Build history of the part. All positions in model axes, mm. Face numbers are marked on the shaded views. Give positions to 0.01 mm unless a question says otherwise; leave off trailing zeros. Order: outer loops, then holes, each group sorted by start corner. A loop starts at its lowest first (then second) coordinate and runs counter-clockwise, first axis right, second up. Notation, with made-up numbers: (74, 16.25) -> (120, 16.25) arc R35 ccw to (120, 49.25) -> close; hole circle Ø8 at (71, -13.5). An arc over 180 degrees is marked (long way). One line per item, written item: value. Start each with the question number.
(1) Probe line 1 (Y direction, x = 4, z = 8); line 2 (X direction, y = 4.55, z = 0); line 3 (X direction, y = -12.6, z = 0). List the from-to ranges inside material, lowest first.
(2) Saw through at C-C on z = 0. Count the separate pieces of the cut face and the enclosed holes in it, plus the area to 3 significant figures.
(3) Pin check, flat tips, straight feed: pin 1 (14.5 mm diameter, centred on x = 0, z = 0, fed in from +Y); pin 2 (14.5 mm diameter, centred on x = -2.5, z = 2, fed in from +Y); pin 3 (1.5 mm diameter, centred on y = -11.5, z = 11, fed in from -X); pin 4 (2 mm diameter, centred on x = -11, y = -11, fed in from +Z). Stop position of each tip, or through.
(4) Two-plate mould, pull along X, no slides. Class the marked faces 1, 2 and 3: +X half, -X half, draft (parallel to the pull), parting line (faces both ways), or undercut.
(5) Saw through at B-B on y = 9.5. Give the cut face in (x, z), plus the area to 3 significant figures.
(6) Saw through at A-A on y = -7.25. Give the cut face in (x, z).
```python
from build123d import *

# Parameters (mm, degrees)
ESBO_O4_W                        = 2.25
ESBO_O4_H                        = 16
F_4_5_4_5_DIAMETER_HOLE2_D       = 4.5
F_4_5_4_5_DIAMETER_HOLE2_DEPTH   = 18
F_4_5_4_5_DIAMETER_HOLE2_TIP     = 1.351936393
ESBO_O12_R                       = 16
ESBO_O12_R_2                     = 9
RESSALTO_EXTRUS_O1_DEPTH         = 1
CHANFRO1_SIZE                    = 0.5
CHANFRO2_SIZE                    = 0.25
FURO_DE_DI_METRO_4_5_4_5_2_D     = 4.5
FURO_DE_DI_METRO_4_5_4_5_2_DEPTH = 8
FURO_DE_DI_METRO_4_5_4_5_2_TIP   = 1.351936393


# Read off the part's stored shape, not the designer's step: PadrãoCircular5
with BuildPart() as part:
    # Esboço1 → Revolução1 (revolve)
    with BuildSketch(Plane.XY, mode=Mode.PRIVATE) as revolu_o1_sk:
        Polygon((3, -14), (16, -14), (16, 10), (8, 10), (8, 8.5), (9, 8.5), (9, 6.5), (8, 6.5), (8, 5), (9.5, 5), (9.5, 3), (9, 3), (9, -3), (9.5, -3), (9.5, -5), (8, -5), (8, -6.5), (9, -6.5), (9, -8.5), (8, -8.5), (8, -10), (3, -10), align=None)
    revolve(revolu_o1_sk.sketch.rotate(Axis((0, -14, 0), (0, 1, 0)), 90), axis=Axis((0, -14, 0), (0, 1, 0)))

    # Esboço4 → Furo de diâmetro Ø4.5 (4.5)1 (revolve, cut)
    with BuildSketch(Plane(origin=(16, 0, 0), x_dir=(0, 0, -1), z_dir=(0, 1, 0))):
        with Locations((1.125, 8)):
            Rectangle(ESBO_O4_W, ESBO_O4_H)
    revolve(axis=Axis((22.35, 0, 0), (-1, 0, 0)), mode=Mode.SUBTRACT)

    # Ø4.5 (4.5) Diameter Hole2
    with Locations(Plane(origin=(-13.856406461, 0, -8), x_dir=(0, -1, 0), z_dir=(-0.8660254037844364, 0, -0.5000000000000041))):
        with Locations((0, 0)):
            Hole(F_4_5_4_5_DIAMETER_HOLE2_D / 2, depth=F_4_5_4_5_DIAMETER_HOLE2_DEPTH)
            with Locations((0, 0, -(F_4_5_4_5_DIAMETER_HOLE2_DEPTH + F_4_5_4_5_DIAMETER_HOLE2_TIP / 2))):  # 118° drill point
                Cone(0, F_4_5_4_5_DIAMETER_HOLE2_D / 2, F_4_5_4_5_DIAMETER_HOLE2_TIP, mode=Mode.SUBTRACT)

    # Esboço12 → Ressalto-extrusão1 (add)
    with BuildSketch(Plane(origin=(0, 10, 0), x_dir=(1, 0, 0), z_dir=(0, 1, 0))):
        with Locations(Location((0, 0, 0), (0, 0, 90))):
            Circle(ESBO_O12_R)
        with Locations(Location((0, 0, 0), (0, 0, 90))):
            Circle(ESBO_O12_R_2, mode=Mode.SUBTRACT)
    extrude(amount=RESSALTO_EXTRUS_O1_DEPTH)

    # Esboço13 → Furo roscado de M3x0.51 (revolve, cut)
    with BuildSketch(Plane(origin=(11.328847338, 11, -5.282728272), x_dir=(0, 0, 1), z_dir=(1, 0, 0))):
        Polygon((0, 0), (0, 10.751075774), (1.25, 10), (1.25, 0), align=None)
    revolve(axis=Axis((11.328847338, 17.35, -5.282728272), (0, -1, 0)), mode=Mode.SUBTRACT)

    # PadrãoCircular5 outline → PadrãoCircular5 (revolve, cut)
    with BuildSketch(Plane(origin=(5.282728272, 0, 11.328847338), x_dir=(1, 0, 0), z_dir=(0, 0, 1))):
        Polygon((0, 11), (0, 0.248924226), (1.25, 1), (1.25, 11), align=None)
    revolve(axis=Axis((5.282728272, 0, 11.328847338), (0, 1, 0)), mode=Mode.SUBTRACT)

    # Padr_oCircular5 2 outline → Padr_oCircular5 2 (revolve, cut)
    with BuildSketch(Plane(origin=(-11.328847338, 0, 5.282728272), x_dir=(1, 0, 0), z_dir=(0, 0, 1))):
        Polygon((0, 11), (0, 0.248924226), (1.25, 1), (1.25, 11), align=None)
    revolve(axis=Axis((-11.328847338, 0, 5.282728272), (0, 1, 0)), mode=Mode.SUBTRACT)

    # Padr_oCircular5 3 outline → Padr_oCircular5 3 (revolve, cut)
    with BuildSketch(Plane(origin=(-5.282728272, 0, -11.328847338), x_dir=(1, 0, 0), z_dir=(0, 0, 1))):
        Polygon((0, 11), (0, 0.248924226), (1.25, 1), (1.25, 11), align=None)
    revolve(axis=Axis((-5.282728272, 0, -11.328847338), (0, 1, 0)), mode=Mode.SUBTRACT)

    # Chanfro1
    chanfro1_edges = [part.edges().sort_by_distance(p)[0] for p in [
        (0, -10, 3),
    ]]
    chamfer(chanfro1_edges, length=CHANFRO1_SIZE)

    # Chanfro2
    chanfro2_edges = [part.edges().sort_by_distance(p)[0] for p in [
        (0, 11, 9),
    ]]
    chamfer(chanfro2_edges, length=CHANFRO2_SIZE)

    # Furo de diâmetro Ø4.5 (4.5)2
    with Locations(Plane(origin=(-16, 0, 0), x_dir=(0, 0, -1), z_dir=(-1, 0, 0))):
        with Locations((0, 0)):
            Hole(FURO_DE_DI_METRO_4_5_4_5_2_D / 2, depth=FURO_DE_DI_METRO_4_5_4_5_2_DEPTH)
            with Locations((0, 0, -(FURO_DE_DI_METRO_4_5_4_5_2_DEPTH + FURO_DE_DI_METRO_4_5_4_5_2_TIP / 2))):  # 118° drill point
                Cone(0, FURO_DE_DI_METRO_4_5_4_5_2_D / 2, FURO_DE_DI_METRO_4_5_4_5_2_TIP, mode=Mode.SUBTRACT)


solid = part.part
```
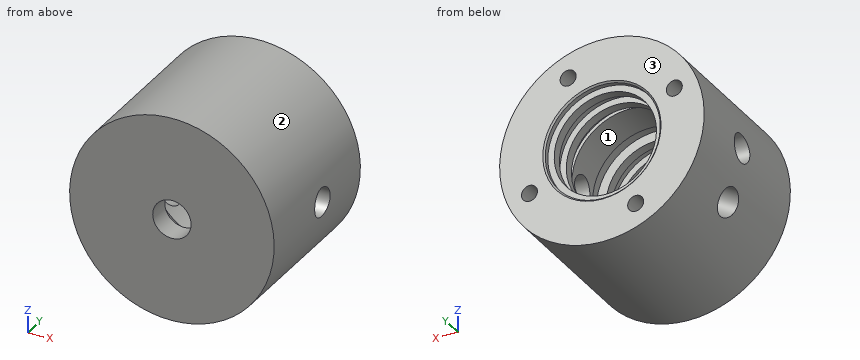
Results below:
1. line 1: y = -14 to -8.5, -6.5 to -5, 5 to 6.5, 8.5 to 10
1. line 2: x = -16 to -9.5, 9.5 to 16
1. line 3: x = -16 to -3, 3 to 16
2. separate pieces: 4
2. enclosed holes: 0
2. area: 343 mm²
3. pin 1: stops at y = -10
3. pin 2: stops at y = 11
3. pin 3: stops at x = -12.29
3. pin 4: stops at z = 12.49
4. face 1: undercut
4. face 2: parting line
4. face 3: draft
5. outline: circle Ø32 at (0, 0); hole circle Ø2.5 at (-11.33, 5.28); hole circle Ø16 at (0, 0); hole circle Ø2.5 at (-5.28, -11.33); hole circle Ø2.5 at (5.28, 11.33); hole circle Ø2.5 at (11.33, -5.28)
5. area: 584 mm²
6. outline: circle Ø32 at (0, 0); hole circle Ø18 at (0, 0)
